For this review, take the finished solid that the model builds, in its own axes (mm). Face numbers are marked on the shaded views. A direction names the side the tool comes from. Give positions to 0.01 mm unless a question says otherwise; leave off trailing zeros. Loops run counter-clockwise (first coordinate to the right, second up) from the corner with the lowest first, then second, coordinate; pieces in that order, holes last.
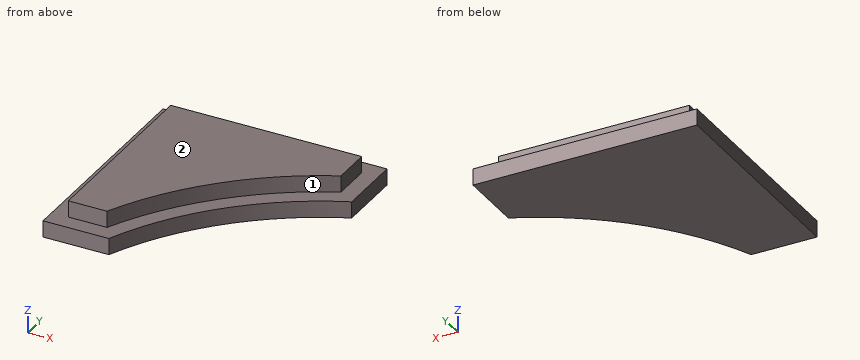
```python
from build123d import *

# Parameters (mm, degrees)
F1_DEPTH = 12.7
F3_DEPTH = 6.35


with BuildPart() as f1:
    # F0 (on Top) → F1 (new body)
    with BuildSketch(Plane.XY):
        with BuildLine():
            Line((-44.3746231037, 130.7346231037), (-130.7346231037, 130.7346231037))
            Line((-130.7346231037, 130.7346231037), (-130.7346231037, 44.3746231037))
            Line((-130.7346231037, 44.3746231037), (-105.3346231037, 44.3746231037))
            ThreePointArc((-105.3346231037, 44.3746231037), (-80.8223050896, 80.8223050896), (-44.3746231037, 105.3346231037))
            Line((-44.3746231037, 105.3346231037), (-44.3746231037, 130.7346231037))
        make_face()
    extrude(amount=F1_DEPTH)

    # F2 (on face) → F3 (cut)
    with BuildSketch(Plane.XY.offset(12.7)):
        with BuildLine():
            Line((-44.3746231037, 130.7346231037), (-130.7346231037, 130.7346231037))
            Line((-130.7346231037, 130.7346231037), (-130.7346231037, 44.3746231037))
            Line((-130.7346231037, 44.3746231037), (-105.3346231037, 44.3746231037))
            ThreePointArc((-105.3346231037, 44.3746231037), (-80.8223050896, 80.8223050896), (-44.3746231037, 105.3346231037))
            Line((-44.3746231037, 105.3346231037), (-44.3746231037, 130.7346231037))
        make_face()
        with BuildLine():
            Line((-124.3846231037, 124.3846231037), (-50.7246231037, 124.3846231037))
            Line((-50.7246231037, 124.3846231037), (-50.7246231037, 109.4650677811))
            ThreePointArc((-50.7246231037, 109.4650677811), (-85.2982218646, 85.2982218646), (-109.4650677811, 50.7246231037))
            Line((-109.4650677811, 50.7246231037), (-124.3846231037, 50.7246231037))
            Line((-124.3846231037, 50.7246231037), (-124.3846231037, 124.3846231037))
        make_face(mode=Mode.SUBTRACT)
    extrude(amount=-F3_DEPTH, mode=Mode.SUBTRACT)


solid = f1.part
```
Item 1: Take a section at A-A on z = 2. Give the boundary of the cut face in (x, y).
Answer:
outline: (-130.73, 44.37) - (-105.33, 44.37) arc R114.3 cw to (-44.37, 105.33) - (-44.37, 130.73) - (-130.73, 130.73) - close
Item 2: Take a section at C-C on x = -74.5. Give the boundary of the cut face in (y, z), and give its area (3 significant figures).
Answer:
outline: (86.68, 0) - (130.73, 0) - (130.73, 6.35) - (124.38, 6.35) - (124.38, 12.7) - (94.88, 12.7) - (94.88, 6.35) - (86.68, 6.35) - close
area: 467 mm2
Item 3: Clearance check with flat-ended pins moving along their axes: pin 1 Ø4 at (x, y) = (-103.5, 85) entering from -Z; pin 2 Ø1.9 at (y, z) = (101.5, 10.5) entering from -X; pin 3 Ø4 at (y, z) = (95.5, 9) entering from +X; pin 4 Ø3 at (x, z) = (-118.5, 8) entering from -Y. State where each tip first meets the part, or that it passes through.
Answer:
pin 1: stops at z = 0
pin 2: stops at x = -124.38
pin 3: stops at x = -71.04
pin 4: stops at y = 50.72
Item 4: Tool access review of the marked faces 1 and 2: name each direction out of +Z, -Z, +X, -X, +Y, -Y from which nothing blocks a thin tool from reaching the whole face with its end or side.
Answer:
face 1: +Z, +X, -Y
face 2: +Z, +X, -X, +Y, -Y
Item 5: Take a section at D-D on z = 8.75. Give the boundary of the cut face in (x, y).
Answer:
outline: (-124.38, 50.72) - (-109.47, 50.72) arc R120.9 cw to (-50.72, 109.47) - (-50.72, 124.38) - (-124.38, 124.38) - close
Item 6: For L1, parallel to Z at x = -125, y = 126; L2, parallel to X at y = 121, z = 10.5; L3, parallel to X at y = 94, z = 10, list the stretches that pass through material, from the lowest coordinate up.
Answer:
L1: z = 0 to 6.35
L2: x = -124.38 to -50.72
L3: x = -124.38 to -75.6
Item 7: Take a section at B-B on y = 115. Give the boundary of the cut face in (x, z), and give its area (3 significant figures).
Answer:
outline: (-130.73, 0) - (-44.37, 0) - (-44.37, 6.35) - (-50.72, 6.35) - (-50.72, 12.7) - (-124.38, 12.7) - (-124.38, 6.35) - (-130.73, 6.35) - close
area: 1,020 mm2
